Autodesk Inventor part; units mm, degrees
ref_plane "YZ Plane" through (0, 0, 0) normal (1, 0, 0) x (0, 1, 0)
ref_plane "XZ Plane" through (0, 0, 0) normal (0, 1, 0) x (-1, 0, 0)
ref_plane "XY Plane" through (0, 0, 0) normal (0, 0, 1) x (1, 0, 0)
sketch "Sketch1" plane through (0, 0, 0) normal (0, 0, 1) x (1, 0, 0)
  line L0 (-15, 0) -> (-125.4596, 0)
  line L1 (-130.9191, 0) -> (-130.9191, 30)
  line L2 (-114.5404, 30) -> (-15, 30)
  line L3 (0, 15) -> (0, 15)
  line L4 (-130.9191, 0) -> (-111.6355, 22.9813)
  line L5 (-111.6355, 22.9813) -> (-120, 30)
  line L6 (-190.2213, 69.3416) -> (-190.2213, 69.3416)
  line L7 (-188.3724, 48.2091) -> (-135.1014, 3.5093)
  line L8 (-124.1823, 33.5093) -> (-169.0888, 71.1904)
  circle A0 centre (-182.5608, 62.9137) radius 5
  circle A1 centre (-10, 15) radius 5
  arc A2 (0, 15) -> (-15, 30) centre (-15, 15) ccw
  arc A3 (-15, 0) -> (0, 15) centre (-15, 15) ccw
  arc A4 (-169.0888, 71.1904) -> (-190.2213, 69.3416) centre (-178.7306, 59.6997) ccw
  arc A5 (-190.2213, 69.3416) -> (-188.3724, 48.2091) centre (-178.7306, 59.6997) ccw
  arc A6 (-124.1823, 33.5093) -> (-114.5404, 30) centre (-114.5404, 45) ccw
  arc A7 (-135.1014, 3.5093) -> (-125.4596, 0) centre (-125.4596, 15) ccw
  line L9 (-15, 15) -> (-82.4661, 15) construction
  line L10 (-178.7306, 59.6997) -> (-70.1019, -31.4506) construction
  circle A8 centre (-125.4596, 15) radius 5
  point P0 (0, 0)
  point P1 (0, 30)
  point P2 (-199.8631, 57.8509)
  point P3 (0, 15)
  point P4 (-190.2213, 69.3416)
  dimension "d0" = 30
  dimension "d2" = 30
  dimension "d3" = 50
  dimension "d4" = 120
  dimension "d5" = 90
  dimension "d6" = 10
  dimension "d7" = 10
  dimension "d8" = 10
  dimension "d9" = 10
  dimension "d10" = 15
  dimension "d13" = 10
  dimension "d14" = 15
  dimension "d15" = 15
extrude "Extrusion1" add sketch "Sketch1" along normal blind 3 contours L0 A7 L7 A5 A4 L8 A6 L2 A2 A3
sketch "Sketch2" plane through (0, 0, 3) normal (0, 0, 1) x (1, 0, 0)
  point P0 (0, 0)
sketch "Sketch3" plane through (0, 0, 3) normal (0, 0, 1) x (1, 0, 0)
  line L0 (-125.4596, 0) -> (-15, 0)
  arc A0 (-15, 0) -> (-15, 30) centre (-15, 15) ccw
  line L1 (-15, 30) -> (-114.5404, 30)
  arc A1 (-124.1823, 33.5093) -> (-114.5404, 30) centre (-114.5404, 45) ccw
  line L2 (-124.1823, 33.5093) -> (-169.0888, 71.1904)
  arc A2 (-169.0888, 71.1904) -> (-188.3724, 48.2091) centre (-178.7306, 59.6997) ccw
  line L3 (-188.3724, 48.2091) -> (-135.1014, 3.5093)
  arc A3 (-135.1014, 3.5093) -> (-125.4596, 0) centre (-125.4596, 15) ccw
  circle A4 centre (-125.4596, 15) radius 5
  circle A5 centre (-10, 15) radius 5
  circle A6 centre (-182.5608, 62.9137) radius 5
  line L4 (-248.5616, 21.4167) -> (-81.5166, 82.2161)
  line L5 (-124.1823, 33.5093) -> (-169.0888, 71.1904)
  point P0 (0, 0)
  point P1 (-151.7599, 56.6497)
  point P2 (-151.7599, 56.6497)
  point P3 (-184.3118, 44.8018)
  dimension "d16" = 60
  dimension "d17" = 36
extrude "Extrusion2" add sketch "Sketch3" along normal blind 3 contours A3 L3 L4 L2 A1 L1 A0 L0
sketch "Sketch4" plane through (0, 0, 0) normal (0, 0, -1) x (-1, 0, 0)
  circle A0 centre (182.5608, 62.9137) radius 5
  point P0 (0, 0)
extrude "Extrusion3" [suppressed]
sketch "Sketch5" plane through (0, 0, 6) normal (0, 0, 1) x (1, 0, 0)
  circle A0 centre (-67.7298, 15) radius 2.5
  circle A1 centre (-10, 15) radius 5
  circle A2 centre (-125.4596, 15) radius 5
  point P0 (0, 0)
  dimension "d22" = 115.4595
  dimension "d23" = 57.7298
  dimension "d28" = 5
extrude "Extrusion4" cut sketch "Sketch5" against normal blind 0.1 contours A0
sketch "Sketch6" plane through (0, 0, 0) normal (0, 0, -1) x (-1, 0, 0)
  circle A0 centre (67.7298, 15) radius 2.5
  point P0 (0, 0)
extrude "Extrusion5" cut sketch "Sketch6" against normal blind 0.1
equation "\"d2\" = d0"
equation "\"d7\" = d6"
equation "\"d8\" = d6"
equation "\"d9\" = d7"
equation "\"d10\" = 0.5 * d0"
equation "\"d13\" = d8"
equation "\"d14\" = 0.5 * d0"
equation "\"d15\" = d14"
equation "\"d18\" = d11"
equation "\"d20\" = 4 * d11"
equation "\"d23\" = 0.5 * d22"
properties part number "GripP1"
Build history of the part. All positions in model axes, mm. A direction names the side the tool comes from. Give positions to 0.01 mm unless a question says otherwise; leave off trailing zeros. Loops run counter-clockwise (first coordinate to the right, second up) from the corner with the lowest first, then second, coordinate; pieces in that order, holes last. Notation, with made-up numbers: (76.25, 58) -> (126.25, 58) arc R28 ccw to (126.25, 93) -> close; hole circle Ø5 at (79.25, -4). An arc over 180 degrees is marked (long way). One line per question, with ' | ' between items.
Q1. Cut at C-C, the plane x = -10. Write the cut outline in (y, z).
Filled sheet:
outline: (0.86, 0) -> (10, 0) -> (10, 6) -> (0.86, 6) -> close; (20, 0) -> (29.14, 0) -> (29.14, 6) -> (20, 6) -> close
Q2. Tool access for faces 1 (the flat face through (-65, 30, 3)), 2 (the flat face through (-168.264, 50.643, 4.479)), 3 (the cylindrical face through (0, 15, 3)): list every direction of +Z, -Z, +X, -X, +Y, -Y with a clear straight run to the whole face (end or side of a thin tool).
Filled sheet:
face 1: +Z, -Z, +X, +Y | face 2: +Z, -X, +Y | face 3: +Z, -Z, +X
Q3. Cut at B-B, the plane y = 15. Write the cut outline in (x, z), plus the area to 3 significant figures.
Filled sheet:
outline: (-148.8, 0) -> (-130.46, 0) -> (-130.46, 6) -> (-148.8, 6) -> close; (-120.46, 0) -> (-70.23, 0) -> (-70.23, 0.1) -> (-65.23, 0.1) -> (-65.23, 0) -> (-15, 0) -> (-15, 6) -> (-65.23, 6) -> (-65.23, 5.9) -> (-70.23, 5.9) -> (-70.23, 6) -> (-120.46, 6) -> close; (-5, 0) -> (0, 0) -> (0, 6) -> (-5, 6) -> close | area: 772 mm²
Q4. Cut at D-D, the plane x = -157. Write the cut outline in (y, z), plus the area to 3 significant figures.
Filled sheet:
outline: (21.88, 0) -> (61.05, 0) -> (61.05, 3) -> (54.74, 3) -> (54.74, 6) -> (21.88, 6) -> close | area: 216 mm²
Q5. Drill centre lines: line 1 along Y through (x, z) = (-67, 2.3); line 2 along X through (y, z) = (13, 4.6); line 3 along X through (y, z) = (61.5, 2). Where is each one in solid material? Low to high. Write a range as [from, to].
Filled sheet:
line 1: y = [0, 30] | line 2: x = [-146.41, -130.04], [-120.88, -14.58], [-5.42, -0.13] | line 3: x = [-193.62, -187.36], [-177.76, -157.54]
Q6. Cut at A-A, the plane z = 4.9. Write the cut outline in (x, y).
Filled sheet:
outline: (-184.31, 44.8) -> (-135.1, 3.51) arc R15 ccw to (-125.46, 0) -> (-15, 0) arc R15 ccw to (-15, 30) -> (-114.54, 30) arc R15 cw to (-124.18, 33.51) -> (-151.76, 56.65) -> close; hole circle Ø10 at (-125.46, 15); hole circle Ø10 at (-10, 15)
Q7. Pull direction X, two halves, no side cores. Call faces 4 (the cylindrical face through (-129.43, 18.04, 2.96)), 5 (the cylindrical face through (-193.66, 58.23, 1.48)), 6 (the flat face through (-141.33, 47.9, 2.96)), 7 (the cylindrical face through (-177.792, 61.412, 1.479)): pulls with the +X half, pulls with the -X half, needs draft (parallel to the pull), parting line crosses it, or undercut.
Filled sheet:
face 4: undercut | face 5: pulls with the -X half | face 6: pulls with the +X half | face 7: undercut
Q8. Drop flat-ended pins along their axis: pin 1 (1.5 mm diameter, centred on x = -68.5, y = 14.5, fed in from +Z); pin 2 (9 mm diameter, centred on x = -162.5, y = 65, fed in from +Z); pin 3 (8 mm diameter, centred on x = -125.46, y = 15, fed in from +Z); pin 4 (1.5 mm diameter, centred on x = -67, y = 14.5, fed in from -Z). Give the stop position or say it passes through.
Filled sheet:
pin 1: stops at z = 5.9 | pin 2: stops at z = 3 | pin 3: passes through | pin 4: stops at z = 0.1
